Read the model definition and answer for the solid it produces. Units are mm, in the model's axes. Face numbers are marked on the shaded views. A direction names the side the tool comes from. Give positions to 0.01 mm unless a question says otherwise; leave off trailing zeros. Write each loop counter-clockwise with the first axis right and the second up, starting at its lowest first coordinate (ties: lowest second). Pieces come first, ordered by that corner, then holes.
Autodesk Inventor part; units mm, degrees
ref_plane "YZ Plane" through (0, 0, 0) normal (1, 0, 0) x (0, 1, 0)
ref_plane "XZ Plane" through (0, 0, 0) normal (0, 1, 0) x (-1, 0, 0)
ref_plane "XY Plane" through (0, 0, 0) normal (0, 0, 1) x (1, 0, 0)
sketch "Esquisse1" plane through (0, 0, 0) normal (0, 1, 0) x (-1, 0, 0)
  line L0 (-20, 20) -> (20, 20)
  line L1 (20, 20) -> (20, -20)
  line L2 (20, -20) -> (-20, -20)
  line L3 (-20, -20) -> (-20, 20)
  line L4 (-20, 20) -> (20, -20) construction
  line L5 (20, 20) -> (-20, -20) construction
  point P0 (0, 0)
  dimension "d0" = 40
  dimension "d1" = 40
extrude "Extrusion1" add sketch "Esquisse1" along normal blind 16
chamfer "Chanfrein1" distance 8 angle 45 4 edges at (-20, 8, 20) (20, 8, 20) (20, 8, -20) (-20, 8, -20)
sketch "Esquisse2" plane through (0, 16, 0) normal (0, 1, 0) x (1, 0, 0)
  line L0 (-20, -20) -> (20, -20)
  line L1 (20, -20) -> (20, 20)
  line L2 (20, 20) -> (-20, 20)
  line L3 (-20, 20) -> (-20, -20)
  line L4 (-20, -20) -> (20, 20) construction
  line L5 (20, -20) -> (-20, 20) construction
  point P0 (0, 0)
  dimension "d7" = 40
extrude "Extrusion2" add sketch "Esquisse2" along normal blind 10
chamfer "Chanfrein2" distance 4 angle 45 4 edges at (20, 21, -20) (20, 21, 20) (-20, 21, 20) (-20, 21, -20)
sketch "Esquisse3" plane through (0, 0, 0) normal (0, -1, 0) x (1, 0, 0)
  line L0 (20, 20) -> (-20, 20)
  line L1 (-20, 20) -> (-20, -20)
  line L2 (-20, -20) -> (20, -20)
  line L3 (20, -20) -> (20, 20)
  line L4 (20, 20) -> (-20, -20) construction
  line L5 (-20, 20) -> (20, -20) construction
  point P0 (0, 0)
  dimension "d13" = 40
  dimension "d14" = 40
extrude "Extrusion3" add sketch "Esquisse3" along normal blind 10
chamfer "Chanfrein3" distance 4 angle 45 4 edges at (-20, -5, 20) (20, -5, 20) (20, -5, -20) (-20, -5, -20)
sketch "Esquisse4" plane through (0, -10, 0) normal (0, -1, 0) x (1, 0, 0)
  circle A0 centre (0, 0) radius 10
  dimension "d20" = 20
extrude "Extrusion4" add sketch "Esquisse4" along normal blind 2
sketch "Esquisse5" plane through (0, -12, 0) normal (0, -1, 0) x (1, 0, 0)
  circle A0 centre (0, 0) radius 1.5
  dimension "d23" = 3
extrude "Extrusion5" add sketch "Esquisse5" along normal blind 18
sketch "Esquisse6" plane through (12, 16, 20) normal (0, 0, 1) x (1, 0, 0)
  line L0 (0, -16) -> (0, 0)
  line L1 (-24, 0) -> (-24, -16)
  line L2 (0, 0) -> (-24, 0)
  line L3 (-28, -16) -> (-24, -16)
  line L4 (0, -16) -> (-24, -16)
  point P0 (-12, -16)
sketch "Esquisse7" plane through (20, 16, -12) normal (1, 0, 0) x (0, 0, -1)
  line L0 (0, 0) -> (-25.6172, 0)
  line L1 (0, -16) -> (-25.6172, -16)
  point P0 (-12, -16)
sketch "Esquisse8" plane through (-12, 16, -20) normal (0, 0, -1) x (-1, 0, 0)
  line L0 (0, 0) -> (0, -16)
  line L1 (-24, -16) -> (-24, 0)
  line L2 (0, 0) -> (-24, 0)
  line L3 (4, -16) -> (0, -16)
  line L4 (0, -16) -> (-24, -16)
  point P0 (-12, -16)
sketch "Esquisse9" plane through (-20, 16, 12) normal (-1, 0, 0) x (0, 0, 1)
  line L0 (0, 0) -> (-24.1988, 0)
  line L1 (0, -16) -> (-24.1988, -16)
  point P0 (-12, -16)
properties part number "Moteur courroie"
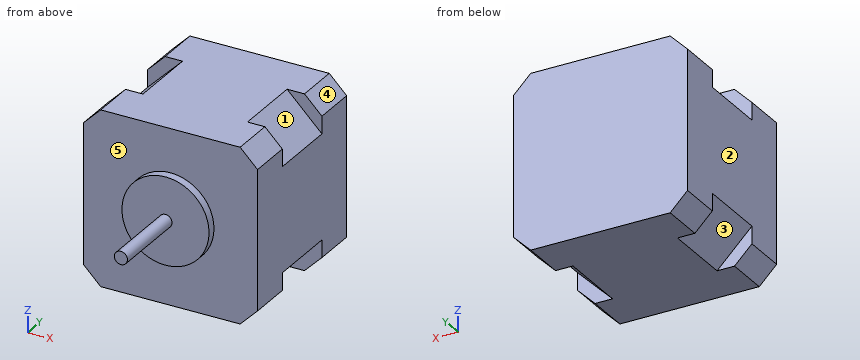
Item 1: Section A-A (x = 0) is taken. Write down the section's boundary in (y, z).
Result set:
outline: (-30, -1.5) - (-12, -1.5) - (-12, -10) - (-10, -10) - (-10, -20) - (26, -20) - (26, 20) - (-10, 20) - (-10, 10) - (-12, 10) - (-12, 1.5) - (-30, 1.5) - close
Item 2: Section B-B (y = 22) is taken. Write down the section's boundary in (x, z).
Result set:
outline: (-20, -16) - (-16, -20) - (16, -20) - (20, -16) - (20, 16) - (16, 20) - (-16, 20) - (-20, 16) - close
Item 3: Each of these flat-tipped pins is pushed along its axis until it touches: pin 1 Ø10 at (x, z) = (-6, 7) entering from -Y; pin 2 Ø3 at (y, z) = (2, 14) entering from -X; pin 3 Ø9 at (x, z) = (16.5, -15.5) entering from -Y. Where does it stop, or does it pass through?
Result set:
pin 1: stops at y = -12
pin 2: stops at x = -19.5
pin 3: stops at y = -10
Item 4: Section D-D (y = 8.5) is taken. Write down the section's boundary in (x, z).
Result set:
outline: (-20, -12) - (-12, -20) - (12, -20) - (20, -12) - (20, 12) - (12, 20) - (-12, 20) - (-20, 12) - close
Item 5: Which of the six approach directions +Z, -Z, +X, -X, +Y, -Y give full straight-line access (tool end or side, diameter ignored) to the marked faces 1 and 2?
Result set:
face 1: +Z, +X
face 2: +Z, -Z, -X, +Y, -Y
Item 6: Determine the mould class of the marked faces 3, 4 and 5 for opening direction Y: pulls with the +Y half, pulls with the -Y half, needs draft (parallel to the pull), parting line crosses it, or undercut.
Result set:
face 3: undercut
face 4: needs draft
face 5: pulls with the -Y half
Item 7: Find the intervals of material crossed by line 1 along Y through (x, z) = (-9.5, -0.5); line 2 along Y through (x, z) = (12.5, 18); line 3 along Z through (x, y) = (-16.5, 8), in increasing order.
Result set:
line 1: y = -12 to 26
line 2: y = -10 to 26
line 3: z = -15.5 to 15.5
Item 8: Section C-C (z = 0) is taken. Write down the section's boundary in (x, y).
Result set:
outline: (-20, -10) - (-10, -10) - (-10, -12) - (-1.5, -12) - (-1.5, -30) - (1.5, -30) - (1.5, -12) - (10, -12) - (10, -10) - (20, -10) - (20, 26) - (-20, 26) - close
